```python
from build123d import *

# Parameters (mm, degrees)
BOSS_EXTRUDE1_DEPTH = 40
SKETCH2_R           = 1.75
CUT_EXTRUDE1_DEPTH  = 40
FILLET1_R           = 3
FILLET2_R           = 20
SKETCH3_R           = 1.6
CUT_EXTRUDE2_DEPTH  = 40
FILLET3_R           = 1.5


with BuildPart() as part:
    # Sketch1 → Boss-Extrude1 (new body)
    with BuildSketch(Plane(origin=(0, 0, 0), x_dir=(0, 0, -1), z_dir=(1, 0, 0))):
        Polygon((0, 0), (40, 0), (40, -1.5), (-1.5, -1.5), (-1.5, 44.5), (0, 44.5), align=None)
    extrude(amount=BOSS_EXTRUDE1_DEPTH)

    # Sketch2 → Cut-Extrude1 (cut)
    with BuildSketch(Plane.XZ.offset(1.5)):
        with Locations(Location((5, -32, 0), (0, 0, 270))):
            Circle(SKETCH2_R)
        with Locations(Location((5, -8, 0), (0, 0, 270))):
            Circle(SKETCH2_R)
        with Locations(Location((35, -8, 0), (0, 0, 270))):
            Circle(SKETCH2_R)
        with Locations(Location((35, -32, 0), (0, 0, 270))):
            Circle(SKETCH2_R)
    extrude(amount=-CUT_EXTRUDE1_DEPTH, mode=Mode.SUBTRACT)

    # Fillet1
    fillet1_edges = [part.edges().sort_by_distance(p)[0] for p in [
        (40, -0.75, -40),
        (0, -0.75, -40),
    ]]
    fillet(fillet1_edges, radius=FILLET1_R)

    # Fillet2
    fillet2_edges = [part.edges().sort_by_distance(p)[0] for p in [
        (40, 44.5, 0.75),
        (0, 44.5, 0.75),
    ]]
    fillet(fillet2_edges, radius=FILLET2_R - 0.0001)  # a hair under: the kernel refuses the full size

    # Sketch3 → Cut-Extrude2 (cut)
    with BuildSketch(Plane.XY.offset(1.5)):
        with Locations((4.5, 24.5)):
            Circle(SKETCH3_R)
        with Locations((12.25, 37.923393759)):
            Circle(SKETCH3_R)
        with Locations((27.75, 37.923393759)):
            Circle(SKETCH3_R)
        with Locations((35.5, 24.5)):
            Circle(SKETCH3_R)
        with Locations((27.75, 11.076606241)):
            Circle(SKETCH3_R)
        with Locations((12.25, 11.076606241)):
            Circle(SKETCH3_R)
        with BuildLine():
            Line((26.5, 31.5), (26.5, 17.5))
            ThreePointArc((26.5, 17.5), (20, 11), (13.5, 17.5))
            Line((13.5, 17.5), (13.5, 31.5))
            ThreePointArc((13.5, 31.5), (20, 38), (26.5, 31.5))
        make_face()
    extrude(amount=-CUT_EXTRUDE2_DEPTH, mode=Mode.SUBTRACT)

    # Fillet3
    fillet3_edges = [part.edges().sort_by_distance(p)[0] for p in [
        (20, 0, 0),
        (20, -1.5, 1.5),
    ]]
    fillet(fillet3_edges, radius=FILLET3_R)


solid = part.part
```
Verification items for the finished model (mm, model axes). A direction names the side the tool comes from. Give positions to 0.01 mm unless a question says otherwise; leave off trailing zeros. Order: outer loops, then holes, each group sorted by start corner. A loop starts at its lowest first (then second) coordinate and runs counter-clockwise, first axis right, second up. Notation, with made-up numbers: (18, 77.5) -> (59, 77.5) arc R7 cw to (59, 81.5) -> close; hole circle Ø5 at (79.5, -10). An arc over 180 degrees is marked (long way). One line per item, written item: value.
(1) Draft check along X on faces 1 (the face through (11.903, 36.361, 0.76)), 2 (the face through (40, -1, -9)), 3 (the face through (29, 19, 0)). Enter one of: pulls with the +X half, pulls with the -X half, needs draft (parallel to the pull), parting line crosses it, or undercut.
Final values:
face 1: undercut
face 2: pulls with the +X half
face 3: needs draft
(2) Sectioned sample at D-D on x = 36. Record the cut outline in (y, z), then the cut area to 3 significant figures.
Final values:
outline: (-1.5, -40) -> (0, -40) -> (0, -33.44) -> (-1.5, -33.44) -> close; (-1.5, -30.56) -> (0, -30.56) -> (0, -9.44) -> (-1.5, -9.44) -> close; (-1.5, -6.56) -> (0, -6.56) -> (0, -1.5) arc R1.5 cw to (1.5, 0) -> (22.98, 0) -> (22.98, 1.5) -> (0, 1.5) arc R1.5 ccw to (-1.5, 0) -> close; (26.02, 0) -> (36.5, 0) -> (36.5, 1.5) -> (26.02, 1.5) -> close
area: 104 mm^2
(3) Tool access check on faces 4 (the face through (20, 11, 1)), 5 (the face through (5.08, -0.76, -30.25)), 6 (the face through (20, 0, -20)). Record the directions out of +Z, -Z, +X, -X, +Y, -Y that give a thin tool (end or side, any length) a straight path to the whole face; none if there is none.
Final values:
face 4: +Z, -Z
face 5: +Y, -Y
face 6: -Z, +X, -X, +Y
(4) Sectioned sample at B-B on y = 19. Record the cut outline in (x, z).
Final values:
outline: (0, 0) -> (13.5, 0) -> (13.5, 1.5) -> (0, 1.5) -> close; (26.5, 0) -> (40, 0) -> (40, 1.5) -> (26.5, 1.5) -> close
(5) Sectioned sample at C-C on x = 12.25. Record the cut outline in (y, z).
Final values:
outline: (-1.5, -40) -> (0, -40) -> (0, -1.5) arc R1.5 cw to (1.5, 0) -> (9.48, 0) -> (9.48, 1.5) -> (0, 1.5) arc R1.5 ccw to (-1.5, 0) -> close; (12.68, 0) -> (36.32, 0) -> (36.32, 1.5) -> (12.68, 1.5) -> close; (39.52, 0) -> (42.94, 0) -> (42.94, 1.5) -> (39.52, 1.5) -> close
(6) Sectioned sample at A-A on z = -8. Record the cut outline in (x, y), then the cut area to 3 significant figures.
Final values:
outline: (0, -1.5) -> (3.25, -1.5) -> (3.25, 0) -> (0, 0) -> close; (6.75, -1.5) -> (33.25, -1.5) -> (33.25, 0) -> (6.75, 0) -> close; (36.75, -1.5) -> (40, -1.5) -> (40, 0) -> (36.75, 0) -> close
area: 49.5 mm^2
(7) Gauge pin test, flat ends, axial feed: pin 1 (6 mm diameter, centred on x = 21.5, y = 24, fed in from -Z); pin 2 (5 mm diameter, centred on x = 27.75, y = 37.92, fed in from -Z); pin 3 (4.5 mm diameter, centred on x = 5, z = -32, fed in from +Y). Record the tip position at first contact, or that the pin passes through.
Final values:
pin 1: through
pin 2: z = 0
pin 3: y = 0
(8) Scan lines: line 1 along X through (y, z) = (-1.05, -8); line 2 along Y through (x, z) = (15, -31); line 3 along Y through (x, z) = (4.5, 0.5). Record each from-to range of solid material in increasing order. Write a range as [from, to].
Final values:
line 1: [0, 3.25], [6.75, 33.25], [36.75, 40]
line 2: [-1.5, 0]
line 3: [-1.41, 22.9], [26.1, 37.14]
